Verification items for the finished model (mm, model axes). A direction names the side the tool comes from. Coordinates: 2 decimals unless noted, no trailing zeros. Order: outer loops, then holes, each group sorted by start corner. A loop starts at its lowest first (then second) coordinate and runs counter-clockwise, first axis right, second up. Notation, with made-up numbers: M 38.25,25 L 70.25,25 A16 ccw 70.25,52 Z; hole C -20.75,70 d9. An arc over 180 degrees is marked long. Return JSON: item names as keys, results as strings.
```python
from build123d import *

# Parameters (mm, degrees)
DIAM_TRE_DU_PER_AGE_0_15_0_15_1_D = 15.9
CHANFREIN1_SIZE                   = 0.5


with BuildPart() as part:
    # Esquisse1 → Révolution1 (revolve)
    with BuildSketch(Plane.XY, mode=Mode.PRIVATE) as r_volution1_sk:
        Polygon((0, 0), (0, 12.5), (2.5, 12.5), (2.5, 10), (14.5, 10), (14.5, 0), align=None)
    revolve(r_volution1_sk.sketch.rotate(Axis((-19.53975326, 0, 0), (1, 0, 0)), 180), axis=Axis((-19.53975326, 0, 0), (1, 0, 0)))

    # Diamètre du perçage Ø0.15 (0.15)1 (through all)
    with Locations(Plane(origin=(14.5, 0, 0), x_dir=(0, 0, -1), z_dir=(1, 0, 0))):
        with Locations((0, 0)):
            Hole(DIAM_TRE_DU_PER_AGE_0_15_0_15_1_D / 2)

    # Chanfrein1
    chanfrein1_edges = [part.edges().sort_by_distance(p)[0] for p in [
        (14.5, 0, -7.95),
        (0, 0, -7.95),
        (14.5, 10, 0),
    ]]
    chamfer(chanfrein1_edges, length=CHANFREIN1_SIZE)


solid = part.part
```
Q1. Draft check along Y on faces 3 (the face through (7.16, -7.76, -1.72)), 4 (the face through (1.268, -11.923, -3.755)), 5 (the face through (2.5, 0.1, -10.2)). Enter one of: pulls with the +Y half, pulls with the -Y half, needs draft (parallel to the pull), parting line crosses it, or undercut.
Values:
{"face 3": "undercut", "face 4": "parting line crosses it", "face 5": "needs draft"}
Q2. Cross-section at D-D, the plane x = 4. Record the boundary of the cut face in (y, z).
Values:
{"outline": "C 0,0 d20; hole C 0,0 d15.9"}
Q3. Material ranges on line 1 along X through (y, z) = (-7.25, 7.5); line 2 along Y through (x, z) = (13.25, 1.5); line 3 along Z through (x, y) = (12.25, 6.75), recorded low to high.
Values:
{"line 1": "0 to 2.5", "line 2": "-9.89 to -7.81, 7.81 to 9.89", "line 3": "-7.38 to -4.2, 4.2 to 7.38"}
Q4. Tool access check on faces 1 (the face through (14.5, 8.5, 1.4)), 2 (the face through (8, 10, 0)). Record the directions out of +Z, -Z, +X, -X, +Y, -Y that give a thin tool (end or side, any length) a straight path to the whole face; none if there is none.
Values:
{"face 1": "+Z, -Z, +X, +Y, -Y", "face 2": "+X"}
Q5. Go/stop test with flat-tipped pins: pin 1 (3 mm diameter, centred on x = 9, y = -6.5, fed in from +Z); pin 2 (3 mm diameter, centred on x = 8.5, y = -1, fed in from -Z); pin 3 (1 mm diameter, centred on x = 9.5, z = 3.5, fed in from -Y). Record where each tip stops, or that it passes through.
Values:
{"pin 1": "z = 8.66", "pin 2": "z = -10", "pin 3": "y = -9.54"}
Q6. Cross-section at C-C, the plane x = 1.75. Record the boundary of the cut face in (y, z), and give its area (3 significant figures).
Values:
{"outline": "C 0,0 d25; hole C 0,0 d15.9", "area": "292 mm^2"}
Q7. Cross-section at A-A, the plane z = 0. Record the boundary of the cut face in (x, y), and give its area (3 significant figures).
Values:
{"outline": "M 0,-12.5 L 2.5,-12.5 L 2.5,-10 L 14,-10 L 14.5,-9.5 L 14.5,-8.45 L 14,-7.95 L 0.5,-7.95 L 0,-8.45 Z; M 0,8.45 L 0.5,7.95 L 14,7.95 L 14.5,8.45 L 14.5,9.5 L 14,10 L 2.5,10 L 2.5,12.5 L 0,12.5 Z", "area": "71.2 mm^2"}
